For this review, take the finished solid that the model builds, in its own axes (mm). Face numbers are marked on the shaded views. A direction names the side the tool comes from. Round coordinates to 2 decimals unless told otherwise and drop trailing zeros. Write each loop counter-clockwise with the first axis right and the second up, starting at its lowest first coordinate (ties: lowest second). Pieces come first, ordered by that corner, then holes. Notation, with made-up numbers: (-37, -35.75) -> (-29, -35.75) arc R22 cw to (-29, 3.25) -> close; hole circle Ø4 at (78, 58). An arc over 180 degrees is marked (long way). Answer in a Markdown table with one row per item.
from build123d import *

# Parameters (mm, degrees)
F0_W      = 110
F0_H      = 44
F1_DEPTH  = 21
F4_W      = 43
F4_H      = 21
F5_DEPTH  = 118
F6_DEPTH  = 10
F7_DEPTH  = 5
F9_T      = -4
F10_DEPTH = 25.4
F8_W      = 5
F8_H      = 10
F11_DEPTH = 254
F12_DEPTH = 25.4
F13_W     = 110
F13_H     = 5.2398111895
F14_DEPTH = 25.4


with BuildPart() as f1:
    # F0 (on Top) → F1 (new body)
    with BuildSketch(Plane.XY):
        Rectangle(F0_W, F0_H)
    extrude(amount=F1_DEPTH)


with BuildPart() as f5:
    # F4 (on offset) → F5 (new body)
    with BuildSketch(Plane.YZ.offset(59)):
        with Locations((0, -5.4130828939)):
            Rectangle(F4_W, F4_H)
    extrude(amount=-F5_DEPTH)

    # F6 (add): a face of the model
    f6_faces = [f5.faces().sort_by_distance(p)[0] for p in [
        (0, 0, 5.0869171061),
    ]]
    extrude(f6_faces, amount=F6_DEPTH)

    # F7 (add): a face of the model
    f7_faces = [f5.faces().sort_by_distance(p)[0] for p in [
        (0, 21.5, -0.4130828939),
    ]]
    extrude(f7_faces, amount=F7_DEPTH)

    # F9
    f9_openings = [f5.faces().sort_by_distance(p)[0] for p in [
        (0, 2.5, -15.913083),
    ]]
    offset(amount=F9_T, openings=f9_openings)

    # F10 (cut): a face of the model
    f10_faces = [f5.faces().sort_by_distance(p)[0] for p in [
        (0, 2.5, 11.0869171061),
    ]]
    extrude(f10_faces, amount=-F10_DEPTH, mode=Mode.SUBTRACT)

    # F8 (on face) → F11 (cut)
    with BuildSketch(Plane.YZ.offset(59)):
        Polygon((0, 5.0869171061), (0, -5.9130828939), (21.5, -5.9130828939), (8.5, 5.0869171061), align=None)
        Polygon((-21.5, -5.9130828939), (-21.5, -15.9130828939), (21.5, -15.9130828939), (21.5, -5.9130828939), (0, -5.9130828939), align=None)
        with Locations((24, -10.9130828939)):
            Rectangle(F8_W, F8_H)
        Polygon((26.5, 15.0869171061), (8.5, 15.0869171061), (21.5, 5.0869171061), (26.5, 5.0869171061), align=None)
        Polygon((-8.5, 5.0869171061), (-21.5, -5.9130828939), (0, -5.9130828939), (0, 5.0869171061), align=None)
        Polygon((-21.5, 15.0869171061), (-21.5, 5.0869171061), (-8.5, 15.0869171061), align=None)
    extrude(amount=-F11_DEPTH, mode=Mode.SUBTRACT)

    # F12 (cut): a face of the model
    f12_faces = [f5.faces().sort_by_distance(p)[0] for p in [
        (0, -17.5, 2.8176863368),
    ]]
    extrude(f12_faces, amount=-F12_DEPTH, mode=Mode.SUBTRACT)

    # F13 (on face) → F14 (cut)
    with BuildSketch(Plane(origin=(0, -6.0549280902, 7.1558241066), x_dir=(1, 0, 0), z_dir=(0, 0.6459422415, -0.7633862854))):
        with Locations((0, 17.6124095592)):
            Rectangle(F13_W, F13_H)
    extrude(amount=-F14_DEPTH, mode=Mode.SUBTRACT)


solid = f5.part
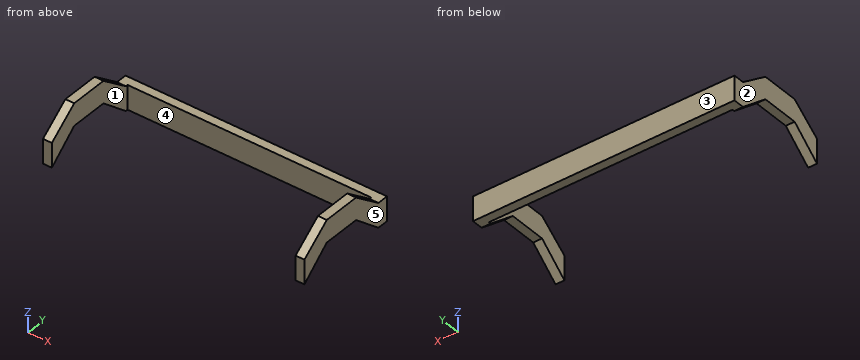
1) For line 1 (X direction, y = -6.5, z = 11.5); line 2 (Y direction, x = -35.5, z = -4.5), list the stretches that pass through material, from the lowest coordinate up. Write a range as [from, to].
Solved:
| item | result |
|---|---|
| line 1 | [-59, -55], [55, 59] |
| line 2 | [22.5, 26.5] |
2) Mouldability with a two-part tool opening along X and no side actions: class the marked faces 3, 4 and 5 as pulls with the +X half, pulls with the -X half, needs draft (parallel to the pull), parting line crosses it, or undercut.
Solved:
| item | result |
|---|---|
| face 3 | needs draft |
| face 4 | undercut |
| face 5 | pulls with the +X half |
3) Consider section D-D on x = -34.5. State the section outline as (y, z) points.
Solved:
| item | result |
|---|---|
| outline | (22.5, -5.91) -> (26.5, -5.91) -> (26.5, 5.09) -> (22.5, 5.09) -> close |
4) Consider section A-A on y = 12.5. State the section outline as (x, z) points.
Solved:
| item | result |
|---|---|
| outline | (-59, 1.7) -> (-55, 1.7) -> (-55, 12.01) -> (-59, 12.01) -> close; (55, 1.7) -> (59, 1.7) -> (59, 12.01) -> (55, 12.01) -> close |
5) Clearance check with flat-ended pins moving along their axes: pin 1 Ø1.5 at (x, z) = (-21.5, -3) entering from -Y; pin 2 Ø1.5 at (x, y) = (25.5, 25) entering from +Z; pin 3 Ø4.5 at (x, y) = (57.5, 0) entering from -Z; pin 4 Ø12 at (x, z) = (44.5, 12.5) entering from +Y. State where each tip first meets the part, or that it passes through.
Solved:
| item | result |
|---|---|
| pin 1 | y = 22.5 |
| pin 2 | z = 5.09 |
| pin 3 | z = 5.09 |
| pin 4 | through |
6) Consider section B-B on z = -0.5. State the section outline as (x, y) points.
Solved:
| item | result |
|---|---|
| outline | (-59, -21.5) -> (-55, -21.5) -> (-55, -15.1) -> (-59, -15.1) -> close; (-59, 15.1) -> (-55, 15.1) -> (-55, 22.5) -> (55, 22.5) -> (55, 15.1) -> (59, 15.1) -> (59, 26.5) -> (-59, 26.5) -> close; (55, -21.5) -> (59, -21.5) -> (59, -15.1) -> (55, -15.1) -> close |
7) Consider section C-C on z = 12.75. State the section outline as (x, y) points.
Solved:
| item | result |
|---|---|
| outline | (-59, -11.54) -> (-55, -11.54) -> (-55, 11.54) -> (-59, 11.54) -> close; (55, -11.54) -> (59, -11.54) -> (59, 11.54) -> (55, 11.54) -> close |
8) For the marked faces 1 and 2, list the 3-axis set-ups (+Z, -Z, +X, -X, +Y, -Y) from which the entire face can be reached by the end or side of a thin tool; tool diameter is ignored.
Solved:
| item | result |
|---|---|
| face 1 | +Z, -Z, -Y |
| face 2 | +Z, -Z, -X, +Y, -Y |
